Input: part model. Units: mm. Frame: model coordinates. Coordinates: 2 decimals unless noted, no trailing zeros. Order: outer loops, then holes, each group sorted by start corner. A loop starts at its lowest first (then second) coordinate and runs counter-clockwise, first axis right, second up. Notation, with made-up numbers: (53, 11) - (64, 11) arc R13 ccw to (64, 15) - close; hole circle Ø9 at (68, 12). An arc over 180 degrees is marked (long way). One line per question, with ' | ' between items.
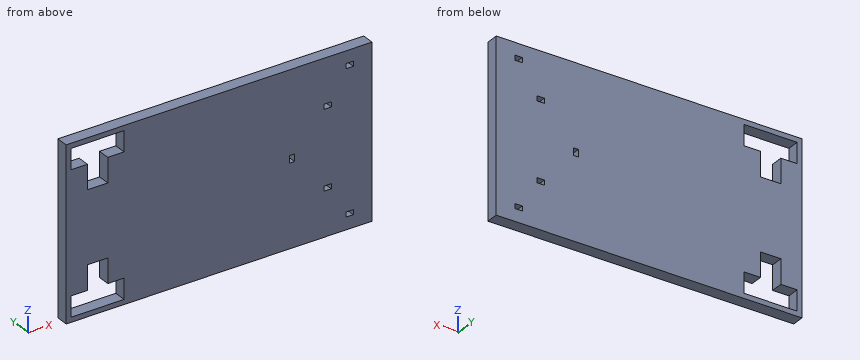
from build123d import *

# Parameters (mm, degrees)
SKETCH1_W           = 375
SKETCH1_H           = 210
BOSS_EXTRUDE1_DEPTH = 15
SKETCH1_5_W         = 25
SKETCH1_5_H         = 30
CUT_EXTRUDE2_DEPTH  = 34
SKETCH1_6_W         = 65
SKETCH1_6_H         = 25
CUT_EXTRUDE3_DEPTH  = 46
SKETCH1_7_W         = 65
SKETCH1_7_H         = 25
CUT_EXTRUDE4_DEPTH  = 48
SKETCH1_8_W         = 25
SKETCH1_8_H         = 30
CUT_EXTRUDE5_DEPTH  = 45
SKETCH1_9_W         = 9
SKETCH1_9_H         = 6
CUT_EXTRUDE6_DEPTH  = 34
SKETCH1_10_W        = 9
SKETCH1_10_H        = 6
CUT_EXTRUDE7_DEPTH  = 31
SKETCH1_11_W        = 6
SKETCH1_11_H        = 9
CUT_EXTRUDE8_DEPTH  = 34
SKETCH1_12_W        = 9
SKETCH1_12_H        = 6
CUT_EXTRUDE9_DEPTH  = 27
SKETCH1_13_W        = 9
SKETCH1_13_H        = 6
CUT_EXTRUDE10_DEPTH = 31


with BuildPart() as part:
    # Sketch1 → Boss-Extrude1 (new body)
    with BuildSketch(Plane(origin=(0, 0, 0), x_dir=(1, 0, 0), z_dir=(0, 1, 0))):
        with Locations((187.5, 105)):
            Rectangle(SKETCH1_W, SKETCH1_H)
    extrude(amount=BOSS_EXTRUDE1_DEPTH)

    # Sketch1<5> → Cut-Extrude2 (cut)
    with BuildSketch(Plane(origin=(0, 0, 0), x_dir=(1, 0, 0), z_dir=(0, 1, 0))):
        with Locations((38.5, 164)):
            Rectangle(SKETCH1_5_W, SKETCH1_5_H)
    extrude(amount=CUT_EXTRUDE2_DEPTH, mode=Mode.SUBTRACT)

    # Sketch1<6> → Cut-Extrude3 (cut)
    with BuildSketch(Plane(origin=(0, 0, 0), x_dir=(1, 0, 0), z_dir=(0, 1, 0))):
        with Locations((38.5, 191.5)):
            Rectangle(SKETCH1_6_W, SKETCH1_6_H)
    extrude(amount=CUT_EXTRUDE3_DEPTH, mode=Mode.SUBTRACT)

    # Sketch1<7> → Cut-Extrude4 (cut)
    with BuildSketch(Plane(origin=(0, 0, 0), x_dir=(1, 0, 0), z_dir=(0, 1, 0))):
        with Locations((38.5, 18.5)):
            Rectangle(SKETCH1_7_W, SKETCH1_7_H)
    extrude(amount=CUT_EXTRUDE4_DEPTH, mode=Mode.SUBTRACT)

    # Sketch1<8> → Cut-Extrude5 (cut)
    with BuildSketch(Plane(origin=(0, 0, 0), x_dir=(1, 0, 0), z_dir=(0, 1, 0))):
        with Locations((38.5, 46)):
            Rectangle(SKETCH1_8_W, SKETCH1_8_H)
    extrude(amount=CUT_EXTRUDE5_DEPTH, mode=Mode.SUBTRACT)

    # Sketch1<9> → Cut-Extrude6 (cut)
    with BuildSketch(Plane(origin=(0, 0, 0), x_dir=(1, 0, 0), z_dir=(0, 1, 0))):
        with Locations((347.5, 18)):
            Rectangle(SKETCH1_9_W, SKETCH1_9_H)
    extrude(amount=CUT_EXTRUDE6_DEPTH, mode=Mode.SUBTRACT)

    # Sketch1<10> → Cut-Extrude7 (cut)
    with BuildSketch(Plane(origin=(0, 0, 0), x_dir=(1, 0, 0), z_dir=(0, 1, 0))):
        with Locations((320.5, 57)):
            Rectangle(SKETCH1_10_W, SKETCH1_10_H)
    extrude(amount=CUT_EXTRUDE7_DEPTH, mode=Mode.SUBTRACT)

    # Sketch1<11> → Cut-Extrude8 (cut)
    with BuildSketch(Plane(origin=(0, 0, 0), x_dir=(1, 0, 0), z_dir=(0, 1, 0))):
        with Locations((277, 105)):
            Rectangle(SKETCH1_11_W, SKETCH1_11_H)
    extrude(amount=CUT_EXTRUDE8_DEPTH, mode=Mode.SUBTRACT)

    # Sketch1<12> → Cut-Extrude9 (cut)
    with BuildSketch(Plane(origin=(0, 0, 0), x_dir=(1, 0, 0), z_dir=(0, 1, 0))):
        with Locations((320.5, 153)):
            Rectangle(SKETCH1_12_W, SKETCH1_12_H)
    extrude(amount=CUT_EXTRUDE9_DEPTH, mode=Mode.SUBTRACT)

    # Sketch1<13> → Cut-Extrude10 (cut)
    with BuildSketch(Plane(origin=(0, 0, 0), x_dir=(1, 0, 0), z_dir=(0, 1, 0))):
        with Locations((347.5, 192)):
            Rectangle(SKETCH1_13_W, SKETCH1_13_H)
    extrude(amount=CUT_EXTRUDE10_DEPTH, mode=Mode.SUBTRACT)


solid = part.part
Item 1: Section A-A on z = -41. Return the cut outline in (x, y).
Data:
outline: (0, 0) - (26, 0) - (26, 15) - (0, 15) - close; (51, 0) - (375, 0) - (375, 15) - (51, 15) - close
Item 2: Contact query for a flat-ended pin moving along its axis: P1, Ø1, axis at y = 8.5, z = -69, coming from the -X side. Output: stop coordinate, or through.
Data:
P1: x = 0
Item 3: Ray query, line 1 (Z direction, x = 22, y = 10.25); line 2 (Z direction, x = 278, y = 4.25); line 3 (X direction, y = 13.25, z = -29). Return the intervals inside material, ascending.
Data:
line 1: -210 to -204, -179 to -31, -6 to 0 | line 2: -210 to -109.5, -100.5 to 0 | line 3: 0 to 6, 71 to 375
Item 4: Section B-B on y = 11.25. Count the separate pieces of the cut face and the enclosed holes in it, and give its area (3 significant figures).
Data:
separate pieces: 1 | enclosed holes: 7 | area: 73,700 mm^2
